For this review, take the finished solid that the model builds, in its own axes (mm). Give positions to 0.01 mm unless a question says otherwise; leave off trailing zeros. Loops run counter-clockwise (first coordinate to the right, second up) from the corner with the lowest first, then second, coordinate; pieces in that order, holes last. Notation, with made-up numbers: (-29, -21.75) - (24, -21.75) arc R34 cw to (24, 12.25) - close; hole circle Ø9 at (51, -3.5). An arc over 180 degrees is marked (long way). Put each result on its own line as item: value. Start each with the question number.
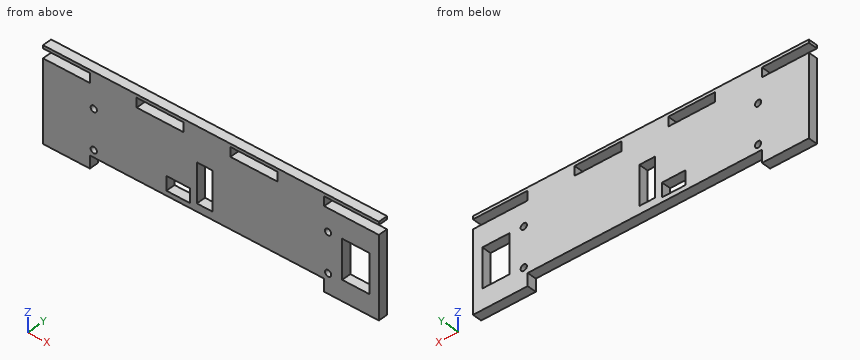
from build123d import *

# Parameters (mm, degrees)
SKETCH_1_W      = 30
SKETCH_1_H      = 6
SKETCH_1_R      = 2
SKETCH_1_W_2    = 10
SKETCH_1_H_2    = 25
SKETCH_1_W_3    = 15
SKETCH_1_H_3    = 9
SKETCH_1_W_4    = 17.5
EXTRUDE_1_DEPTH = 6


with BuildPart() as part:
    # Эскиз1 → Бобышка-Вытянуть1 (new body)
    with BuildSketch(Plane(origin=(0, 0, 0), x_dir=(1, 0, 0), z_dir=(0, 1, 0))):
        Polygon((-77.5, 25), (-107.5, 25), (-107.5, -27), (-77.5, -27), (-77.5, -33), (-107.5, -33), (-107.5, -35), (107.5, -35), (107.5, -33), (72.5, -33), (72.5, -27), (107.5, -27), (107.5, 25), (72.5, 25), (72.5, 17), (-77.5, 17), align=None)
        with Locations((-32.5, -30)):
            Rectangle(SKETCH_1_W, SKETCH_1_H, mode=Mode.SUBTRACT)
        with Locations(Location((-75, -12.5, 0), (0, 0, 270))):
            Circle(SKETCH_1_R, mode=Mode.SUBTRACT)
        with Locations((27.5, -30)):
            Rectangle(SKETCH_1_W, SKETCH_1_H, mode=Mode.SUBTRACT)
        with Locations(Location((75, -12.5, 0), (0, 0, 270))):
            Circle(SKETCH_1_R, mode=Mode.SUBTRACT)
        with Locations((-4, -0.5)):
            Rectangle(SKETCH_1_W_2, SKETCH_1_H_2, mode=Mode.SUBTRACT)
        with Locations((-21, 9.5)):
            Rectangle(SKETCH_1_W_3, SKETCH_1_H_3, mode=Mode.SUBTRACT)
        with Locations(Location((-75, 12.5, 0), (0, 0, 270))):
            Circle(SKETCH_1_R, mode=Mode.SUBTRACT)
        with Locations((92.75, -0.5)):
            Rectangle(SKETCH_1_W_4, SKETCH_1_H_2, mode=Mode.SUBTRACT)
        with Locations(Location((75, 12.5, 0), (0, 0, 270))):
            Circle(SKETCH_1_R, mode=Mode.SUBTRACT)
    extrude(amount=EXTRUDE_1_DEPTH)


solid = part.part
1) Take a section at A-A on x = -75. State the section outline as (y, z) points.
2) Wall thickness on probe 1 along X at (y, z) = (4.9, -1); probe 2 along X at (y, z) = (1.7, -12.5); probe 3 along X at (y, z) = (0.35, 30): over which ranges is each line inside the solid? List them lowest first.
3) Take a section at C-C on y = 2.85. State how many separate pieces and enclosed holes the cut face has, and give its area (3 significant figures).
4) Take a section at B-B on x = 75. State the section outline as (y, z) points.
5) Insertion check: P1, Ø2, axis at x = 10.5, y = 3, coming from the -Z side. The pin has a flat end and moves straight along its axis. Give the tip position at first contact, or say it passes through.
Answers follow:
1. outline: (0, -17) - (6, -17) - (6, -14.5) - (0, -14.5) - close; (0, -10.5) - (6, -10.5) - (6, 10.5) - (0, 10.5) - close; (0, 14.5) - (6, 14.5) - (6, 35) - (0, 35) - close
2. probe 1: -107.5 to -9, 1 to 84, 101.5 to 107.5
2. probe 2: -107.5 to -77, -73 to -28.5, -13.5 to 73, 77 to 107.5
2. probe 3: -77.5 to -47.5, -17.5 to 12.5, 42.5 to 72.5
3. separate pieces: 1
3. enclosed holes: 9
3. area: 10,100 mm2
4. outline: (0, -25) - (6, -25) - (6, -14.5) - (0, -14.5) - close; (0, -10.5) - (6, -10.5) - (6, 10.5) - (0, 10.5) - close; (0, 14.5) - (6, 14.5) - (6, 27) - (0, 27) - close; (0, 33) - (6, 33) - (6, 35) - (0, 35) - close
5. P1: z = -17
